from build123d import *

# Parameters (mm, degrees)
F1_DEPTH = 30
F3_D     = 4.3
F3_DEPTH = 10


with BuildPart() as f1:
    # F0 (on Top) → F1 (new body)
    with BuildSketch(Plane.XY):
        Polygon((45.5, 26), (-45.5, 26), (-45.5, -26), (-38.5, -26), (-38.5, 19), (38.5, 19), (38.5, -26), (45.5, -26), align=None)
    extrude(amount=F1_DEPTH)

    # F3
    with Locations(Plane(origin=(-45.5, 0, 0), x_dir=(0, -1, 0), z_dir=(-1, 0, 0))):
        with Locations((-4, 15)):
            Hole(F3_D / 2, depth=F3_DEPTH)


solid = f1.part
Design review of the part built by this model. Coordinates are the model's own, in mm. A direction names the side the tool comes from. Round coordinates to 2 decimals unless told otherwise and drop trailing zeros. Write each loop counter-clockwise with the first axis right and the second up, starting at its lowest first coordinate (ties: lowest second). Pieces come first, ordered by that corner, then holes.
Item 1: Consider section B-B on y = 4. Give the boundary of the cut face in (x, z).
Item 2: For pin 1 Ø15 at (x, z) = (12, 15) entering from -Y, flat-tipped, find the tip position at first contact; note if it passes through.
Item 3: Consider section C-C on y = -10.5. Give the boundary of the cut face in (x, z), and give its area (3 significant figures).
Item 4: Consider section A-A on z = 15. Give the boundary of the cut face in (x, y), and give its area (3 significant figures).
Item 5: Wall thickness on L1, parallel to X at y = -22, z = 12; L2, parallel to Z at x = -39.75, y = 4; L3, parallel to Y at x = 15, z = 16.75: over which ranges is each line inside the solid? List them lowest first.
Item 6: Draft analysis for pull direction X (two halves, no side actions). For faces 3 (the flat face through (-1, 19, 15)), 4 (the flat face through (45.5, 0, 15)), 5 (the cylindrical face through (-41.95, 3.53, 12.9)), state which applies: released by +X, released by -X, zero draft, split by the parting line, or undercut.
Item 7: For faces 1 (the flat face through (-42, -26, 15)), 2 (the flat face through (-38.5, -4, 15)), list the 3-axis set-ups (+Z, -Z, +X, -X, +Y, -Y) from which the entire face can be reached by the end or side of a thin tool; tool diameter is ignored.
Item 8: Consider section D-D on z = 27.5. Give the boundary of the cut face in (x, y), and give its area (3 significant figures).
Check values:
1. outline: (-45.5, 0) - (-38.5, 0) - (-38.5, 12.85) - (-45.5, 12.85) - close; (-45.5, 17.15) - (-38.5, 17.15) - (-38.5, 30) - (-45.5, 30) - close; (38.5, 0) - (45.5, 0) - (45.5, 30) - (38.5, 30) - close
2. pin 1: stops at y = 19
3. outline: (-45.5, 0) - (-38.5, 0) - (-38.5, 30) - (-45.5, 30) - close; (38.5, 0) - (45.5, 0) - (45.5, 30) - (38.5, 30) - close
3. area: 420 mm2
4. outline: (-45.5, -26) - (-38.5, -26) - (-38.5, 1.85) - (-45.5, 1.85) - close; (-45.5, 6.15) - (-38.5, 6.15) - (-38.5, 19) - (38.5, 19) - (38.5, -26) - (45.5, -26) - (45.5, 26) - (-45.5, 26) - close
4. area: 1,240 mm2
5. L1: x = -45.5 to -38.5, 38.5 to 45.5
5. L2: z = 0 to 12.85, 17.15 to 30
5. L3: y = 19 to 26
6. face 3: undercut
6. face 4: released by +X
6. face 5: zero draft
7. face 1: +Z, -Z, +X, -X, -Y
7. face 2: +Z, -Z, -Y
8. outline: (-45.5, -26) - (-38.5, -26) - (-38.5, 19) - (38.5, 19) - (38.5, -26) - (45.5, -26) - (45.5, 26) - (-45.5, 26) - close
8. area: 1,270 mm2
